Part model, mm, in its own coordinate system. A direction names the side the tool comes from. Give positions to 0.01 mm unless a question says otherwise; leave off trailing zeros. Order: outer loops, then holes, each group sorted by start corner. A loop starts at its lowest first (then second) coordinate and runs counter-clockwise, first axis right, second up. Notation, with made-up numbers: M 56,23 L 65,23 A30 ccw 65,48 Z; hole C -34,-37 d7. An arc over 180 degrees is marked long. Answer as a JSON object with one key per item and string values.
from build123d import *

# Parameters (mm, degrees)
EXTRUDE_1_DEPTH     = 1100
SKETCH_2_R          = 7.5
CUT_EXTRUDE_1_DEPTH = 61


with BuildPart() as part:
    # Эскиз1 → Вытянуть-Тонкостенный1 (new body)
    with BuildSketch(Plane(origin=(0, 0, 0), x_dir=(1, 0, 0), z_dir=(0, 1, 0))):
        with BuildLine():
            Line((-25, 30), (25, 30))
            ThreePointArc((25, 30), (28.535533906, 28.535533906), (30, 25))
            Line((30, 25), (30, -25))
            ThreePointArc((30, -25), (28.535533906, -28.535533906), (25, -30))
            Line((25, -30), (-25, -30))
            ThreePointArc((-25, -30), (-28.535533906, -28.535533906), (-30, -25))
            Line((-30, -25), (-30, 25))
            ThreePointArc((-30, 25), (-28.535533906, 28.535533906), (-25, 30))
        make_face()
        with BuildLine():
            Line((-25, 27), (25, 27))
            ThreePointArc((25, 27), (26.414213562, 26.414213562), (27, 25))
            Line((27, 25), (27, -25))
            ThreePointArc((27, -25), (26.414213562, -26.414213562), (25, -27))
            Line((25, -27), (-25, -27))
            ThreePointArc((-25, -27), (-26.414213562, -26.414213562), (-27, -25))
            Line((-27, -25), (-27, 25))
            ThreePointArc((-27, 25), (-26.414213562, 26.414213562), (-25, 27))
        make_face(mode=Mode.SUBTRACT)
    extrude(amount=EXTRUDE_1_DEPTH)

    # Эскиз2 → Вырез-Вытянуть1 (cut, through all)
    with BuildSketch(Plane(origin=(30, 0, 0), x_dir=(0, 0, -1), z_dir=(1, 0, 0))):
        with Locations((0, 25)):
            Circle(SKETCH_2_R)
    extrude(amount=-CUT_EXTRUDE_1_DEPTH, mode=Mode.SUBTRACT)


solid = part.part
1. Which spindle directions (+Z, -Z, +X, -X, +Y, -Y) get a long thin tool onto all of the face, cutting with end or side? Do faces 5 (the flat face through (-27, 542, 0)), 6 (the flat face through (-30, 542, 0)). Say none if no direction does.
Worked answers:
{"face 5": "+Y, -Y", "face 6": "+Z, -Z, -X, +Y, -Y"}
2. Cut at A-A on y = 960.5. Give the cut face in (x, z).
Worked answers:
{"outline": "M -30,-25 A5 ccw -25,-30 L 25,-30 A5 ccw 30,-25 L 30,25 A5 ccw 25,30 L -25,30 A5 ccw -30,25 Z; hole M -27,-25 A2 ccw -25,-27 L 25,-27 A2 ccw 27,-25 L 27,25 A2 ccw 25,27 L -25,27 A2 ccw -27,25 Z"}
3. Two-plate mould, pull along Z, no slides. Class faces 1 (the flat face through (0, 542, -27)), 2 (the flat face through (27, 542, 0)), 3 (the flat face through (0, 542, 30)), 4 (the flat face through (0, 542, -30)): +Z half, -Z half, draft (parallel to the pull), parting line (faces both ways), or undercut.
Worked answers:
{"face 1": "undercut", "face 2": "undercut", "face 3": "+Z half", "face 4": "-Z half"}
4. Probe line 1 along Z through (x, y) = (-12, 685.5); line 2 along Y through (x, z) = (-28, 0). List the from-to ranges inside material, lowest first.
Worked answers:
{"line 1": "z = -30 to -27, 27 to 30", "line 2": "y = 0 to 17.5, 32.5 to 1100"}
